Here's how the part is built. I have some questions about the finished solid (model axes, mm). A direction names the side the tool comes from. Round coordinates to 2 decimals unless told otherwise and drop trailing zeros. Loops run counter-clockwise (first coordinate to the right, second up) from the corner with the lowest first, then second, coordinate; pieces in that order, holes last. Notation, with made-up numbers: (-37.5, -11.75) -> (-24.5, -11.75) arc R28 cw to (-24.5, 27.25) -> close; hole circle Ø3 at (63.5, -5.5). An arc over 180 degrees is marked (long way). Use one line per item in the form item = value. Start each with the question number.
Item 1: If we section it at B-B (z = -9.25): Write out the boundary of the cut face in (x, y).
Item 2: For faces 1 (the face through (-1.94, 3.93, 3.79)), 2 (the face through (-3.5, 3, 7)), which set-ups out of +Z, -Z, +X, -X, +Y, -Y let a thin tool reach every point of the face, with its end or its side?
Item 3: I'm going to push flat-ended pins straight in: pin 1 Ø1.2 at (y, z) = (2.5, 7) entering from -X; pin 2 Ø0.6 at (x, y) = (-0.5, 5) entering from -Z; pin 3 Ø3 at (y, z) = (4.5, -7.5) entering from +X. Where does each tip first touch, or does it pass through?
Item 4: Thinking about a two-plate mould opening in Y: for faces 3 (the face through (0, 6, -3)), 4 (the face through (0, 0, -3)), 5 (the face through (-0.89, 4.957, 10.466)), 6 (the face through (0, 5.5, 1.85)), which applies, released by +Y, released by -Y, zero draft, split by the parting line, or undercut?
Item 5: If we section it at A-A (z = 4): Write out the boundary of the cut face in (x, y), then the cut area to 3 significant figures.
Item 6: If I drill on L1, parallel to X at y = 4.5, z = 5; L2, parallel to X at y = 5.75, z = 2; L3, parallel to Z at x = -1.5, y = 4.75 (3 decimals), over which ranges is the centre line in solid material (lowest first)? Write a range as [from, to].
Item 7: If we section it at D-D (x = -8.25): Write out the boundary of the cut face in (y, z), then the cut area to 3 significant figures.
Item 8: If we section it at C-C (y = 1.5): Write out the boundary of the cut face in (x, z) (3 decimals).
```python
from build123d import *

# Parameters (mm, degrees)
SKETCH1_R               = 12.5
BOSS_EXTRUDE1_DEPTH     = 6
CUT_EXTRUDE1_REACH      = 20.668
CUT_EXTRUDE2_REACH      = 20.668
SKETCH3_W               = 7
SKETCH3_H               = 2.4
CUT_EXTRUDE3_DEPTH      = 1
CUT_EXTRUDE3_DEPTH_BACK = 20.954260197
SKETCH4_R               = 2.15
SKETCH5_R               = 2.65
CUT_EXTRUDE4_DEPTH      = 19.668154869


with BuildPart() as part:
    # Sketch1 → Boss-Extrude1 (new body)
    with BuildSketch(Plane(origin=(0, 0, 0), x_dir=(1, 0, 0), z_dir=(0, 1, 0))):
        with Locations(Location((0, 0, 0), (0, 0, 270))):
            Circle(SKETCH1_R)
    extrude(amount=BOSS_EXTRUDE1_DEPTH)

    # Sketch2 → Cut-Extrude1 (cut, up to next)
    with BuildSketch(Plane(origin=(0, 6, 0), x_dir=(1, 0, 0), z_dir=(0, 1, 0)), mode=Mode.PRIVATE) as cut_extrude1_sk1:
        with BuildLine():
            ThreePointArc((0, 2.65), (-2.441823089, 1.029563014), (-1.897366596, -1.85))
            Line((-1.897366596, -1.85), (0, -1.85))
            Line((0, -1.85), (0, 2.65))
        make_face()
    cut_extrude1_tool1 = extrude(cut_extrude1_sk1.sketch, amount=-CUT_EXTRUDE1_REACH, mode=Mode.PRIVATE) & part.part
    # Sketch2 → Cut-Extrude1 (cut, up to next)
    with BuildSketch(Plane(origin=(0, 6, 0), x_dir=(1, 0, 0), z_dir=(0, 1, 0)), mode=Mode.PRIVATE) as cut_extrude1_sk2:
        with BuildLine():
            Line((0, 2.65), (0, -1.85))
            Line((0, -1.85), (1.897366596, -1.85))
            ThreePointArc((1.897366596, -1.85), (2.454640654, -0.998618676), (2.65, 0))
            ThreePointArc((2.65, 0), (1.87383297, 1.87383297), (0, 2.65))
        make_face()
    cut_extrude1_tool2 = extrude(cut_extrude1_sk2.sketch, amount=-CUT_EXTRUDE1_REACH, mode=Mode.PRIVATE) & part.part
    # Sketch2 → Cut-Extrude1 (cut, up to next)
    with BuildSketch(Plane(origin=(0, 6, 0), x_dir=(1, 0, 0), z_dir=(0, 1, 0)), mode=Mode.PRIVATE) as cut_extrude1_sk3:
        with BuildLine():
            ThreePointArc((0, 2.65), (-2.441823089, 1.029563014), (-1.897366596, -1.85))
            Line((-1.897366596, -1.85), (0, -1.85))
            Line((0, -1.85), (0, 2.65))
        make_face()
    cut_extrude1_tool3 = extrude(cut_extrude1_sk3.sketch, amount=-CUT_EXTRUDE1_REACH, mode=Mode.PRIVATE) & part.part
    # Sketch2 → Cut-Extrude1 (cut, up to next)
    with BuildSketch(Plane(origin=(0, 6, 0), x_dir=(1, 0, 0), z_dir=(0, 1, 0)), mode=Mode.PRIVATE) as cut_extrude1_sk4:
        with BuildLine():
            Line((0, 2.65), (0, -1.85))
            Line((0, -1.85), (1.897366596, -1.85))
            ThreePointArc((1.897366596, -1.85), (2.454640654, -0.998618676), (2.65, 0))
            ThreePointArc((2.65, 0), (1.87383297, 1.87383297), (0, 2.65))
        make_face()
    cut_extrude1_tool4 = extrude(cut_extrude1_sk4.sketch, amount=-CUT_EXTRUDE1_REACH, mode=Mode.PRIVATE) & part.part
    add(cut_extrude1_tool1.solids().sort_by_distance((-1.166256, 6, -0.228052))[0], mode=Mode.SUBTRACT)
    add(cut_extrude1_tool2.solids().sort_by_distance((1.166256, 6, -0.228052))[0], mode=Mode.SUBTRACT)
    add(cut_extrude1_tool3.solids().sort_by_distance((-1.166256, 6, -0.228052))[0], mode=Mode.SUBTRACT)
    add(cut_extrude1_tool4.solids().sort_by_distance((1.166256, 6, -0.228052))[0], mode=Mode.SUBTRACT)

    # Sketch3 → Cut-Extrude2 (cut, up to next)
    with BuildSketch(Plane(origin=(0, 6, 0), x_dir=(1, 0, 0), z_dir=(0, 1, 0)), mode=Mode.PRIVATE) as cut_extrude2_sk1:
        with Locations((0, -7.175)):
            Rectangle(SKETCH3_W, SKETCH3_H)
    cut_extrude2_tool1 = extrude(cut_extrude2_sk1.sketch, amount=-CUT_EXTRUDE2_REACH, mode=Mode.PRIVATE) & part.part
    add(cut_extrude2_tool1.solids().sort_by_distance((0, 6, 7.175))[0], mode=Mode.SUBTRACT)

    # Sketch4 → Cut-Extrude3 (cut, two sides: drawn at the far end of the back side and taken through both)
    with BuildSketch(Plane(origin=(0, 0, 1.85), x_dir=(-1, 0, 0), z_dir=(0, 0, -1)).offset(-CUT_EXTRUDE3_DEPTH_BACK)):
        with Locations(Location((0, 3, 0), (0, 0, 208.05505294))):
            Circle(SKETCH4_R)
    extrude(amount=CUT_EXTRUDE3_DEPTH + CUT_EXTRUDE3_DEPTH_BACK, mode=Mode.SUBTRACT)

    # Sketch5 → Cut-Extrude4 (cut, through all)
    with BuildSketch(Plane(origin=(0, 6, 0), x_dir=(1, 0, 0), z_dir=(0, 1, 0))):
        with Locations(Location((0, 8, 0), (0, 0, 270))):
            Circle(SKETCH5_R)
        with Locations(Location((6.92820323, -4, 0), (0, 0, 270))):
            Circle(SKETCH5_R)
        with Locations(Location((-6.92820323, -4, 0), (0, 0, 270))):
            Circle(SKETCH5_R)
    extrude(amount=-CUT_EXTRUDE4_DEPTH, mode=Mode.SUBTRACT)


solid = part.part
```
Values found:
q1.outline = (-8.41, 0) -> (-2.34, 0) -> (-2.34, 6) -> (-8.41, 6) -> close; (2.34, 0) -> (8.41, 0) -> (8.41, 6) -> (2.34, 6) -> close
q2.face_1 = +Z
q2.face_2 = +Y, -Y
q3.pin_1 = -10.74
q3.pin_2 = -12.5
q3.pin_3 = 10.97
q4.face_3 = released by +Y
q4.face_4 = released by -Y
q4.face_5 = undercut
q4.face_6 = zero draft
q5.outline = (-11.84, 0) -> (-9.58, 0) -> (-9.58, 6) -> (-11.84, 6) -> close; (-4.28, 0) -> (4.28, 0) -> (4.28, 6) -> (-4.28, 6) -> close; (9.58, 0) -> (11.84, 0) -> (11.84, 6) -> (9.58, 6) -> close; hole circle Ø4.3 at (0, 3)
q5.area = 64.0 mm2
q6.L1 = [-11.46, -9.38], [-4.47, -1.54], [1.54, 4.47], [9.38, 11.46]
q6.L2 = [-12.34, -8.67], [-5.19, 5.19], [8.67, 12.34]
q6.L3 = [-12.41, -10.185], [-5.815, -2.185], [1.85, 5.975], [8.375, 12.41]
q7.outline = (0, -9.39) -> (6, -9.39) -> (6, 1.7) -> (0, 1.7) -> close; (0, 6.3) -> (6, 6.3) -> (6, 9.39) -> (0, 9.39) -> close
q7.area = 85.1 mm2
q8.outline = (-3.5, 5.975) -> (-3.5, 8.375) -> (-1.54, 8.375) -> (-1.54, 12.405) arc R12.5 ccw (long way) to (1.54, 12.405) -> (1.54, 8.375) -> (3.5, 8.375) -> (3.5, 5.975) -> (1.54, 5.975) -> (1.54, 1.85) -> (1.897, 1.85) arc R2.65 cw (long way) to (-1.897, 1.85) -> (-1.54, 1.85) -> (-1.54, 5.975) -> close; hole circle Ø5.3 at (-6.928, 4); hole circle Ø5.3 at (0, -8); hole circle Ø5.3 at (6.928, 4)
